Input: dimensioned drawing with shaded views. Units: mm. Origin: part minimum x, y, z. Give positions to 0.01 mm unless a question says otherwise; leave off trailing zeros. Loops run counter-clockwise (first coordinate to the right, second up) from the corner with the lowest first, then second, coordinate; pieces in that order, holes last. Notation, with made-up numbers: M 32,-6 L 66,-6 A12 cw 66,10 Z; hole C 57,65.25 d1. An arc over 180 degrees is marked long. Answer in a Markdown table with one row per item.
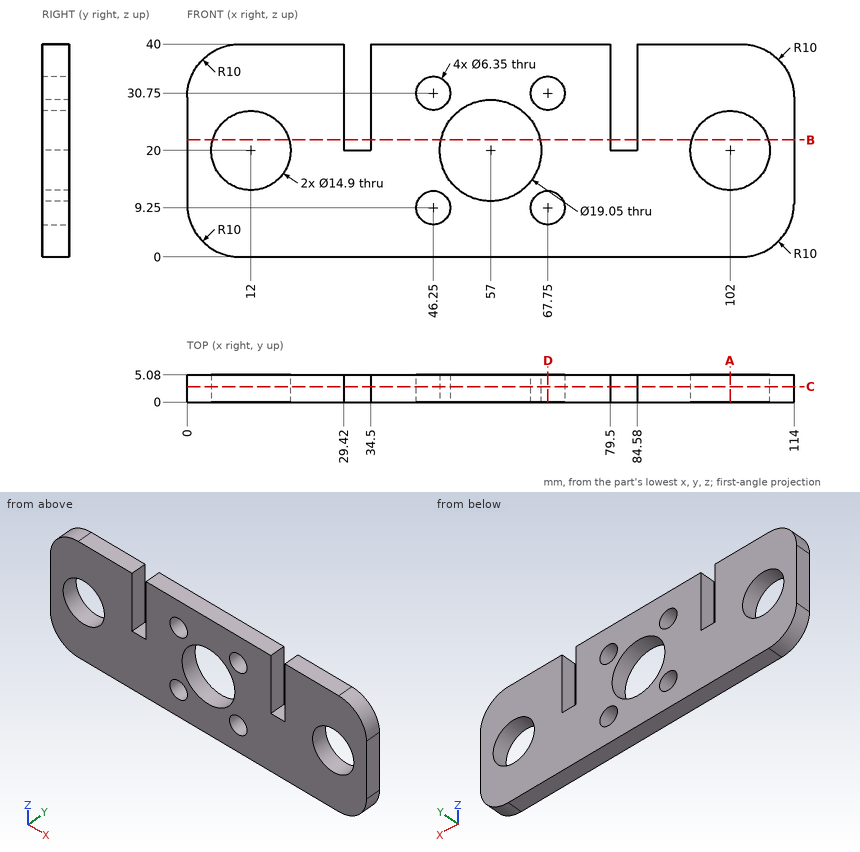
Q1. Section query A-A (x = 102). Output: boundary loops of the cut face in (y, z).
Values follow:
| item | result |
|---|---|
| outline | M 0,0 L 5.08,0 L 5.08,12.55 L 0,12.55 Z; M 0,27.45 L 5.08,27.45 L 5.08,40 L 0,40 Z |
Q2. Section query D-D (x = 67.75). Output: boundary loops of the cut face in (y, z) (3 decimals).
Values follow:
| item | result |
|---|---|
| outline | M 0,0 L 5.08,0 L 5.08,6.075 L 0,6.075 Z; M 0,12.425 L 5.08,12.425 L 5.08,27.575 L 0,27.575 Z; M 0,33.925 L 5.08,33.925 L 5.08,40 L 0,40 Z |
Q3. Contact query for flat-ended pins moving along their axis: pin 1 Ø2.5 at (x, y) = (82.5, 3) entering from +Z; pin 2 Ø2.5 at (y, z) = (2.5, 33.5) entering from +X. Output: stop coordinate, or through.
Values follow:
| item | result |
|---|---|
| pin 1 | z = 20 |
| pin 2 | x = 113.74 |
Q4. Ray query, probe 1 along Z at (x, y) = (46.25, 4.05) (3 decimals); probe 2 along X at (y, z) = (3.8, 9.5); probe 3 along Z at (x, y) = (48.5, 1.4). Return the intervals inside material, ascending. Write a range as from..to.
Values follow:
| item | result |
|---|---|
| probe 1 | 0..6.075, 12.425..27.575, 33.925..40 |
| probe 2 | 0.01..43.08, 49.42..64.58, 70.92..113.99 |
| probe 3 | 0..7.01, 11.49..15.7, 24.3..28.51, 32.99..40 |
Q5. Section query C-C (y = 2.9). Output: boundary loops of the cut face in (x, z) (3 decimals).
Values follow:
| item | result |
|---|---|
| outline | M 0,10 A10 ccw 10,0 L 104,0 A10 ccw 114,10 L 114,30 A10 ccw 104,40 L 84.58,40 L 84.58,20 L 79.5,20 L 79.5,40 L 34.5,40 L 34.5,20 L 29.42,20 L 29.42,40 L 10,40 A10 ccw 0,30 Z; hole C 12,20 d14.9; hole C 46.25,9.25 d6.35; hole C 46.25,30.75 d6.35; hole C 57,20 d19.05; hole C 67.75,9.25 d6.35; hole C 67.75,30.75 d6.35; hole C 102,20 d14.9 |
Q6. Section query B-B (z = 22). Output: boundary loops of the cut face in (x, y).
Values follow:
| item | result |
|---|---|
| outline | M 0,0 L 4.82,0 L 4.82,5.08 L 0,5.08 Z; M 19.18,0 L 29.42,0 L 29.42,5.08 L 19.18,5.08 Z; M 34.5,0 L 47.69,0 L 47.69,5.08 L 34.5,5.08 Z; M 66.31,0 L 79.5,0 L 79.5,5.08 L 66.31,5.08 Z; M 84.58,0 L 94.82,0 L 94.82,5.08 L 84.58,5.08 Z; M 109.18,0 L 114,0 L 114,5.08 L 109.18,5.08 Z |
